Input: part model. Units: mm. Frame: model coordinates. Face numbers are marked on the shaded views. A direction names the side the tool comes from. Round coordinates to 2 decimals unless told otherwise and drop trailing zeros. Loops run counter-clockwise (first coordinate to the right, second up) from the corner with the lowest first, then second, coordinate; pieces in that order, holes last. Notation, with made-up numbers: (72.25, 5) -> (92.25, 5) arc R31 cw to (92.25, 31) -> close; hole circle Ø1 at (-30, 86). An arc over 180 degrees is marked (long way). Answer as a JSON object with one key per item and string values.
```python
from build123d import *

# Parameters (mm, degrees)
PAD_DEPTH       = 20
POCKET_DEPTH    = 15
PAD001_DEPTH    = 8.5
SKETCH005_R     = 3.2
POCKET001_DEPTH = 12.5


with BuildPart() as part:
    # Sketch002 → Pad (new body)
    with BuildSketch(Plane.XY):
        Polygon((8, -7), (8, -27), (10.75, -29.75), (7.993292, -32.5), (-7.924012, -32.5), (-10.75, -29.75), (-8, -27), (-8, -7), align=None)
    extrude(amount=PAD_DEPTH)

    # Sketch004 → Pocket (cut, symmetric)
    with BuildSketch(Plane.YZ):
        Polygon((-29.75, 11.5), (-29.75, 8.5), (-33.75, 4.5), (-33.75, 15.5), align=None)
    extrude(amount=POCKET_DEPTH, both=True, mode=Mode.SUBTRACT)

    # Sketch → Pad001 (join, symmetric)
    with BuildSketch(Plane.YZ):
        with BuildLine():
            ThreePointArc((5.5, 21.489125), (-5.5, 10), (5.5, -1.489125))
            Line((5.5, -1.489125), (5.5, -15))
            Line((5.5, -15), (-7, -15))
            Line((-7, -15), (-7, 35))
            Line((-7, 35), (5.5, 35))
            Line((5.5, 35), (5.5, 21.489125))
        make_face()
    extrude(amount=PAD001_DEPTH, both=True)

    # Sketch005 → Pocket001 (cut, symmetric)
    with BuildSketch(Plane.XZ):
        with Locations((0, 27.5)):
            Circle(SKETCH005_R)
        with Locations((0, -7.5)):
            Circle(SKETCH005_R)
    extrude(amount=POCKET001_DEPTH, both=True, mode=Mode.SUBTRACT)


solid = part.part
```
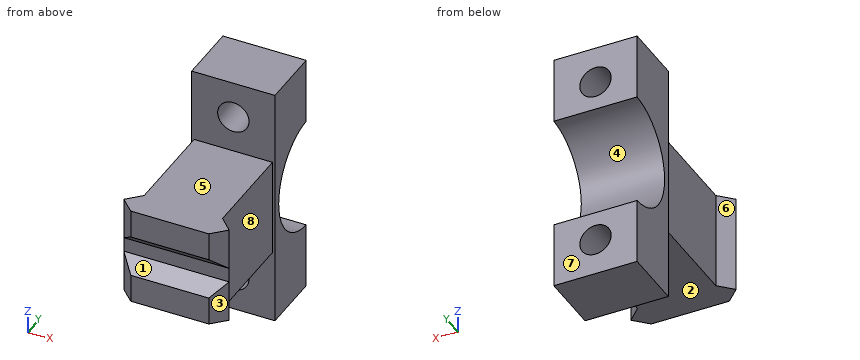
1) Ray query, probe 1 along Z at (x, y) = (0, -0.5); probe 2 along Z at (x, y) = (0, 2.5); probe 3 along X at (y, z) = (-1, 27.5). Return the intervals inside material, ascending.
Output:
{"probe 1": "z = -15 to -10.7, -4.3 to 0.51, 19.49 to 24.3, 30.7 to 35", "probe 2": "z = -15 to -10.7, -4.3 to -0.95, 20.95 to 24.3, 30.7 to 35", "probe 3": "x = -8.5 to -3.2, 3.2 to 8.5"}
2) Section A-A, the plane x = 0. Output: boundary loops of the cut face in (y, z), plus the area to 3 significant figures.
Output:
{"outline": "(-32.5, 0) -> (-7, 0) -> (-7, -4.3) -> (5.5, -4.3) -> (5.5, -1.49) arc R11.5 cw to (5.5, 21.49) -> (5.5, 24.3) -> (-7, 24.3) -> (-7, 20) -> (-32.5, 20) -> (-32.5, 14.25) -> (-29.75, 11.5) -> (-29.75, 8.5) -> (-32.5, 5.75) -> close; (-7, -15) -> (5.5, -15) -> (5.5, -10.7) -> (-7, -10.7) -> close; (-7, 30.7) -> (5.5, 30.7) -> (5.5, 35) -> (-7, 35) -> close", "area": "763 mm^2"}
3) Section C-C, the plane y = -3. Output: boundary loops of the cut face in (x, z), plus the area to 3 significant figures.
Output:
{"outline": "(-8.5, -15) -> (8.5, -15) -> (8.5, 2.84) -> (-8.5, 2.84) -> close; (-8.5, 17.16) -> (8.5, 17.16) -> (8.5, 35) -> (-8.5, 35) -> close; hole circle Ø6.4 at (0, -7.5); hole circle Ø6.4 at (0, 27.5)", "area": "542 mm^2"}
4) Contact query for flat-ended pins moving along their axis: P1, Ø4, axis at y = -2, z = 17.5, coming from the -X side; P2, Ø16, axis at y = -17, z = 7.5, coming from the +X side; P3, Ø4, axis at x = -5.5, z = 11, coming from the +Y side. Output: stop coordinate, or through.
Output:
{"P1": "stops at x = -8.5", "P2": "stops at x = 8", "P3": "stops at y = -5.1"}
5) Reachability of the marked faces 5, 6, 7 and 8 from +Z, -Z, +X, -X, +Y, -Y: full face, straight path, thin tool, end or side. Return the list, or none.
Output:
{"face 5": "+Z, +X, -X, -Y", "face 6": "+Z, -Z, -X", "face 7": "+Z, -Z, +X, -X, +Y", "face 8": "+Z, -Z, +X"}
6) Section D-D, the plane x = 4.25. Output: boundary loops of the cut face in (y, z), plus the area to 3 significant figures.
Output:
{"outline": "(-32.5, 0) -> (-7, 0) -> (-7, -15) -> (5.5, -15) -> (5.5, -1.49) arc R11.5 cw to (5.5, 21.49) -> (5.5, 35) -> (-7, 35) -> (-7, 20) -> (-32.5, 20) -> (-32.5, 14.25) -> (-29.75, 11.5) -> (-29.75, 8.5) -> (-32.5, 5.75) -> close", "area": "923 mm^2"}
7) Draft query along Z for the marked faces 1, 2, 3 and 4. Return one class per face: +Z half, -Z half, draft (parallel to the pull), parting line (faces both ways), or undercut.
Output:
{"face 1": "undercut", "face 2": "-Z half", "face 3": "draft", "face 4": "undercut"}
8) Section B-B, the plane z = -7.5. Output: boundary loops of the cut face in (x, y).
Output:
{"outline": "(-8.5, -7) -> (-3.2, -7) -> (-3.2, 5.5) -> (-8.5, 5.5) -> close; (3.2, -7) -> (8.5, -7) -> (8.5, 5.5) -> (3.2, 5.5) -> close"}
